Build history of the part. All positions in model axes, mm. Round coordinates to 2 decimals unless told otherwise and drop trailing zeros. Order: outer loops, then holes, each group sorted by start corner. A loop starts at its lowest first (then second) coordinate and runs counter-clockwise, first axis right, second up. Notation, with made-up numbers: M -24,-2 L 1,-2 A13 ccw 1,19 Z; hole C -16.75,41.5 d6. An arc over 180 degrees is marked long. Use CSV: the item, a comma, the result in double quotes.
Autodesk Inventor part; units mm, degrees
ref_plane "YZ Plane" through (0, 0, 0) normal (1, 0, 0) x (0, 1, 0)
ref_plane "XZ Plane" through (0, 0, 0) normal (0, 1, 0) x (-1, 0, 0)
ref_plane "XY Plane" through (0, 0, 0) normal (0, 0, 1) x (1, 0, 0)
sketch "スケッチ1" plane through (0, 0, 0) normal (0, 0, 1) x (1, 0, 0)
  line L0 (0, 0) -> (38, 0)
  line L1 (38, 0) -> (38, 32)
  line L2 (38, 32) -> (0, 32)
  line L3 (0, 32) -> (0, 0)
  dimension "d0" = 38
  dimension "d1" = 32
extrude "押し出し1" add sketch "スケッチ1" along normal blind 4
sketch "スケッチ2" plane through (0, 0, 4) normal (0, 0, 1) x (1, 0, 0)
  line L0 (0, 0) -> (38, 0)
  line L1 (0, 32) -> (0, 0)
  point P0 (4, 4)
  point P1 (4, 28)
  point P2 (34, 4)
  point P3 (34, 28)
  dimension "d4" = 4
  dimension "d5" = 4
  dimension "d8" = 24
  dimension "d11" = 30
hole "穴1" at (4, 4, 4) at (4, 28, 4) at (34, 4, 4) at (34, 28, 4) direction (0, 0, -1) diameter 4.5 end through all
sketch "スケッチ3" plane through (0, 0, 4) normal (0, 0, 1) x (1, 0, 0)
  line L0 (0, 32) -> (0, 0)
  line L1 (0, 16) -> (4, 16)
  line L2 (34, 16) -> (38, 16)
  line L3 (38, 0) -> (38, 32)
  line L4 (4, 16) -> (34, 16)
  dimension "d28" = 30
hole "穴2" at (4, 16, 4) at (34, 16, 4) direction (0, 0, -1) diameter 4.5 depth 4
properties part number "RD004_スペーサ" material "ナイロン 6/6"
(1) Cut at C-C, the plane z = 2.2. Give the cut face in (x, y).
Answer block:
outline,"M 0,0 L 38,0 L 38,32 L 0,32 Z; hole C 4,4 d4.5; hole C 4,16 d4.5; hole C 4,28 d4.5; hole C 34,4 d4.5; hole C 34,16 d4.5; hole C 34,28 d4.5"
(2) Two-plate mould, pull along X, no slides. Class faces 1 (the face through (3.324, 25.854, 1.972)), 2 (the face through (0, 16, 2)), 3 (the face through (19, 16, 4)): released by +X, released by -X, zero draft, split by the parting line, or undercut.
Answer block:
face 1,"undercut"
face 2,"released by -X"
face 3,"zero draft"
(3) Wall check: line 1 (X direction, y = 16, z = 0.95); line 2 (Y direction, x = 34, z = 2.15); line 3 (X direction, y = 5.5, z = 3.75). Give the ranges that are in metal, low to high. Write a range as from..to.
Answer block:
line 1,"x = 0..1.75, 6.25..31.75, 36.25..38"
line 2,"y = 0..1.75, 6.25..13.75, 18.25..25.75, 30.25..32"
line 3,"x = 0..2.32, 5.68..32.32, 35.68..38"
(4) Cut at A-A, the plane x = 34. Give the cut face in (y, z).
Answer block:
outline,"M 0,0 L 1.75,0 L 1.75,4 L 0,4 Z; M 6.25,0 L 13.75,0 L 13.75,4 L 6.25,4 Z; M 18.25,0 L 25.75,0 L 25.75,4 L 18.25,4 Z; M 30.25,0 L 32,0 L 32,4 L 30.25,4 Z"
(5) Cut at D-D, the plane y = 17. Give the cut face in (x, z).
Answer block:
outline,"M 0,0 L 1.98,0 L 1.98,4 L 0,4 Z; M 6.02,0 L 31.98,0 L 31.98,4 L 6.02,4 Z; M 36.02,0 L 38,0 L 38,4 L 36.02,4 Z"
(6) Cut at B-B, the plane y = 28. Give the cut face in (x, z), and give its area (3 significant figures).
Answer block:
outline,"M 0,0 L 1.75,0 L 1.75,4 L 0,4 Z; M 6.25,0 L 31.75,0 L 31.75,4 L 6.25,4 Z; M 36.25,0 L 38,0 L 38,4 L 36.25,4 Z"
area,"116 mm²"
